Read the model definition and answer for the solid it produces. Units are mm, in the model's axes. Face numbers are marked on the shaded views. A direction names the side the tool comes from. Give positions to 0.01 mm unless a question says otherwise; leave off trailing zeros. Write each loop counter-clockwise with the first axis right and the second up, starting at its lowest first coordinate (ties: lowest second). Pieces come first, ordered by that corner, then holes. Notation, with made-up numbers: (-40, 65.25) -> (-33, 65.25) arc R30 cw to (-33, 101.25) -> close; hole circle Ø10 at (27.5, 6.25). An arc over 180 degrees is marked (long way). Use a Markdown table: item, result.
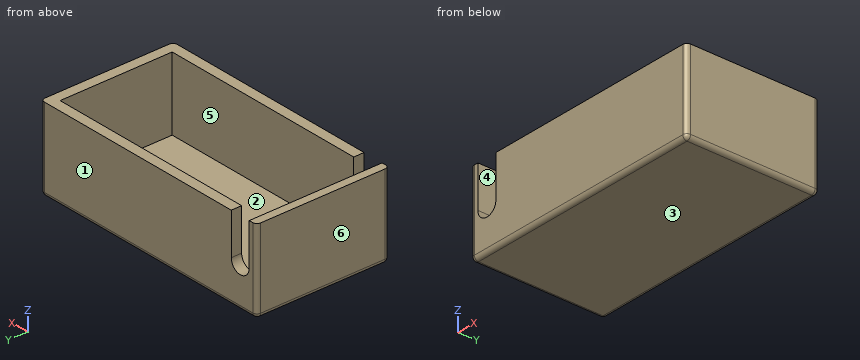
from build123d import *

# Parameters (mm, degrees)
F0_W     = 60
F0_H     = 32
F1_DEPTH = 20
F2_T     = -2.5
F4_DEPTH = 32.001
F5_R     = 1


with BuildPart() as f1:
    # F0 (on Top) → F1 (new body)
    with BuildSketch(Plane.XY):
        Rectangle(F0_W, F0_H)
    extrude(amount=F1_DEPTH)

    # F2
    f2_openings = [f1.faces().sort_by_distance(p)[0] for p in [
        (0, 0, 20),
    ]]
    offset(amount=F2_T, openings=f2_openings)

    # F3 (on face) → F4 (cut, through all)
    with BuildSketch(Plane(origin=(0, 16, 0), x_dir=(-1, 0, 0), z_dir=(0, 1, 0))):
        with BuildLine():
            Line((23, 20), (23, 10))
            ThreePointArc((23, 10), (25.5, 7.5), (28, 10))
            Line((28, 10), (28, 20))
            Line((28, 20), (23, 20))
        make_face()
    extrude(amount=-F4_DEPTH, mode=Mode.SUBTRACT)

    # F5
    f5_edges = [f1.edges().sort_by_distance(p)[0] for p in [
        (30, -16, 10),
        (0, -16, 0),
        (30, 16, 10),
        (30, 0, 0),
        (-30, -16, 10),
        (-30, 16, 10),
        (-30, 0, 0),
        (0, 16, 0),
    ]]
    fillet(f5_edges, radius=F5_R)


solid = f1.part
Item 1: For a pull along Y with two mould halves and no side action, classify the marked faces 1, 2 and 3 as +Y half, -Y half, draft (parallel to the pull), parting line (faces both ways), or undercut.
Return value:
| item | result |
|---|---|
| face 1 | +Y half |
| face 2 | undercut |
| face 3 | draft |
Item 2: A tool of negligible diameter and unlimited length cuts with its end or side. For the marked faces 4, 5 and 6, from which of +Z, -Z, +X, -X, +Y, -Y can it reach the whole face along a straight path? Write none if from no direction.
Return value:
| item | result |
|---|---|
| face 4 | +Z, +Y, -Y |
| face 5 | +Z |
| face 6 | +Z, -Z, -X, +Y, -Y |
Item 3: A cutting plane is placed at D-D (x = -25.5). Give the vertices of the cut face in (y, z).
Return value:
| item | result |
|---|---|
| outline | (-16, 1) arc R1 ccw to (-15, 0) -> (15, 0) arc R1 ccw to (16, 1) -> (16, 7.5) -> (13.5, 7.5) -> (13.5, 2.5) -> (-13.5, 2.5) -> (-13.5, 7.5) -> (-16, 7.5) -> close |
Item 4: A cutting plane is placed at B-B (x = 2.5). Give the vertices of the cut face in (y, z).
Return value:
| item | result |
|---|---|
| outline | (-16, 1) arc R1 ccw to (-15, 0) -> (15, 0) arc R1 ccw to (16, 1) -> (16, 20) -> (13.5, 20) -> (13.5, 2.5) -> (-13.5, 2.5) -> (-13.5, 20) -> (-16, 20) -> close |
Item 5: Straight lines are drawn through the part: line 1 along X through (y, z) = (-1.5, 4); line 2 along Y through (x, z) = (-6.5, 6); line 3 along X through (y, z) = (14.5, 15.25). For each, find the intervals that lie inside material, in ascending order. Write a range as [from, to].
Return value:
| item | result |
|---|---|
| line 1 | [-30, -27.5], [27.5, 30] |
| line 2 | [-16, -13.5], [13.5, 16] |
| line 3 | [-30, -28], [-23, 30] |
Item 6: A cutting plane is placed at C-C (y = -10.5). Give the vertices of the cut face in (x, z), then the cut area to 3 significant figures.
Return value:
| item | result |
|---|---|
| outline | (-30, 1) arc R1 ccw to (-29, 0) -> (29, 0) arc R1 ccw to (30, 1) -> (30, 20) -> (27.5, 20) -> (27.5, 2.5) -> (-27.5, 2.5) -> (-27.5, 8.5) arc R2.5 cw to (-28, 10) -> (-28, 20) -> (-30, 20) -> close |
| area | 232 mm^2 |
Item 7: A cutting plane is placed at A-A (z = 16.25). Give the vertices of the cut face in (x, y).
Return value:
| item | result |
|---|---|
| outline | (-30, -15) arc R1 ccw to (-29, -16) -> (-28, -16) -> (-28, 16) -> (-29, 16) arc R1 ccw to (-30, 15) -> close; (-23, -16) -> (29, -16) arc R1 ccw to (30, -15) -> (30, 15) arc R1 ccw to (29, 16) -> (-23, 16) -> (-23, 13.5) -> (27.5, 13.5) -> (27.5, -13.5) -> (-23, -13.5) -> close |
Item 8: This flat-tipped pin is pushed along its axis until it touches: P1, Ø1.5, axis at x = -0.5, y = 7.5, coming from the +Z side. Where does it stop, or does it pass through?
Return value:
| item | result |
|---|---|
| P1 | z = 2.5 |
